Could you check a few things on this model? Use its own coordinates, in mm. A direction names the side the tool comes from. Coordinates: 2 decimals unless noted, no trailing zeros. Write each loop counter-clockwise with the first axis right and the second up, starting at its lowest first coordinate (ties: lowest second). Pieces come first, ordered by that corner, then holes.
Item 1: If I drill on probe 1 along Z at (x, y) = (0, 4.7); probe 2 along Z at (x, y) = (0, 6.45); probe 3 along X at (y, z) = (2.5, 12.5), over which ranges is the centre line in solid material (lowest first)?
Item 2: I want a section at B-B on y = 1.5. Please give me the cut outline in (x, z).
Item 3: I want a section at A-A on x = 13.5. Please give me the cut outline in (y, z), then the cut area to 3 significant figures.
Item 4: Thinking about a two-plate mould opening in Z: for faces 1 (the flat face through (0, 0, 6)), 2 (the cylindrical face through (23, 6, 0)), 3 (the cylindrical face through (18.5, 3.7, 2.4)), which applies, +Z half, -Z half, draft (parallel to the pull), parting line (faces both ways), or undercut?
Item 5: I want a section at D-D on x = 2.5. Please give me the cut outline in (y, z).
Item 6: For P1, Ø3, axis at x = 10.5, y = 1.5, coming from the +Z side; P2, Ø4, axis at x = 6, y = 5, coming from the +Z side; P3, Ø2, axis at x = -15, z = 17.5, coming from the +Y side; P4, Ø4, axis at x = 13, z = 8, coming from the -Y side, each with a flat end and sliding along its axis, tell me the tip position at first contact or that it passes through.
Item 7: I want a section at C-C on z = 4.5. Please give me the cut outline in (x, y).
Item 8: Which directions (+Z, -Z, +X, -X, +Y, -Y) give clear straight access to the entire face, cutting with the end or side of a thin tool? Please do faces 4 (the flat face through (24, 3.75, 2)), 5 (the flat face through (0, 4, -5)), 6 (the flat face through (13, 6.5, 8)), 7 (the flat face through (-24, 3.75, 2)).
from build123d import *

# Parameters (mm, degrees)
SZKIC2_R                    = 7.5
SZKIC2_R_2                  = 2.4
DODANIE_WYCI_GNI_CIE1_DEPTH = 3.75
SZKIC3_R                    = 5
DODANIE_WYCI_GNI_CIE2_DEPTH = 3.75
SZKIC9_R                    = 7.5
WYTNIJ_WYCI_GNI_CIE3_DEPTH  = 5
SZKIC10_R                   = 2.5
WYTNIJ_WYCI_GNI_CIE4_DEPTH  = 6.5


with BuildPart() as part:
    # Szkic2 → Dodanie-wyciągnięcie1 (new body)
    with BuildSketch(Plane(origin=(0, 0, 0), x_dir=(1, 0, 0), z_dir=(0, 1, 0))):
        with BuildLine():
            Line((-16, 5), (16, 5))
            ThreePointArc((16, 5), (24.235849057, -1.575471698), (17.660377358, -9.811320755))
            ThreePointArc((17.660377358, -9.811320755), (14.373605639, -12.807619738), (10, -12))
            Line((10, -12), (10, -14))
            ThreePointArc((10, -14), (0, -24), (-10, -14))
            Line((-10, -14), (-10, -12.057627201))
            ThreePointArc((-10, -12.057627201), (-14.369651741, -12.856788302), (-17.67794965, -9.892386213))
            ThreePointArc((-17.67794965, -9.892386213), (-24.285167931, -1.607218282), (-16, 5))
        make_face()
        with Locations(Location((0, -14, 0), (0, 0, 270))):
            Circle(SZKIC2_R, mode=Mode.SUBTRACT)
        with Locations(Location((-13, -8, 0), (0, 0, 270))):
            Circle(SZKIC2_R_2, mode=Mode.SUBTRACT)
        with Locations(Location((13, -8, 0), (0, 0, 270))):
            Circle(SZKIC2_R_2, mode=Mode.SUBTRACT)
        with BuildLine():
            Line((-16, 0), (16, 0))
            ThreePointArc((16, 0), (18.5, -2.5), (16, -5))
            Line((16, -5), (-16, -5))
            ThreePointArc((-16, -5), (-18.5, -2.5), (-16, 0))
        make_face(mode=Mode.SUBTRACT)
    extrude(amount=DODANIE_WYCI_GNI_CIE1_DEPTH)

    # Szkic3 → Dodanie-wyciągnięcie2 (add)
    with BuildSketch(Plane(origin=(0, 3.75, 0), x_dir=(1, 0, 0), z_dir=(0, 1, 0))):
        with BuildLine():
            Line((-16, 5), (16, 5))
            ThreePointArc((16, 5), (22.873192437, 0.342120663), (21.093817027, -7.76777683))
            Line((21.093817027, -7.76777683), (6.968542539, -21.17212764))
            ThreePointArc((6.968542539, -21.17212764), (0, -23.952289066), (-6.968542539, -21.17212764))
            Line((-6.968542539, -21.17212764), (-21.093817027, -7.76777683))
            ThreePointArc((-21.093817027, -7.76777683), (-22.873192437, 0.342120663), (-16, 5))
        make_face()
        with Locations(Location((0, -13.8, 0), (0, 0, 270))):
            Circle(SZKIC3_R, mode=Mode.SUBTRACT)
        with BuildLine():
            Line((-16, 0), (16, 0))
            ThreePointArc((16, 0), (18.5, -2.5), (16, -5))
            Line((16, -5), (-16, -5))
            ThreePointArc((-16, -5), (-18.5, -2.5), (-16, 0))
        make_face(mode=Mode.SUBTRACT)
    extrude(amount=DODANIE_WYCI_GNI_CIE2_DEPTH)

    # Szkic9 → Wytnij-wyciągnięcie3 (cut)
    with BuildSketch(Plane.XZ):
        with Locations(Location((0, 14, 0), (0, 0, 270))):
            Circle(SZKIC9_R)
    extrude(amount=-WYTNIJ_WYCI_GNI_CIE3_DEPTH, mode=Mode.SUBTRACT)

    # Szkic10 → Wytnij-wyciągnięcie4 (cut)
    with BuildSketch(Plane.XZ):
        with Locations(Location((-13, 8, 0), (0, 0, 270))):
            Circle(SZKIC10_R)
        with Locations(Location((13, 8, 0), (0, 0, 270))):
            Circle(SZKIC10_R)
    extrude(amount=-WYTNIJ_WYCI_GNI_CIE4_DEPTH, mode=Mode.SUBTRACT)


solid = part.part
Response values:
1. probe 1: z = -5 to 0, 5 to 6.5, 21.5 to 23.95
1. probe 2: z = -5 to 0, 5 to 8.8, 18.8 to 23.95
1. probe 3: x = -15.28 to -10.72, -10 to -7.35, 7.35 to 10, 10.82 to 15.18
2. outline: (-17.68, 9.89) arc R7.49 ccw to (-16, -5) - (16, -5) arc R7.45 ccw to (17.66, 9.81) arc R5 ccw to (10, 12) - (10, 14) arc R10 ccw to (-10, 14) - (-10, 12.06) arc R5.05 ccw to start; hole (-16, 0) - (16, 0) arc R2.5 ccw to (16, 5) - (-16, 5) arc R2.5 ccw to start; hole circle Ø5 at (-13, 8); hole circle Ø15 at (0, 14); hole circle Ø5 at (13, 8)
3. outline: (0, -5) - (7.5, -5) - (7.5, 0) - (0, 0) - close; (0, 5) - (7.5, 5) - (7.5, 14.97) - (3.75, 14.97) - (3.75, 12.97) - (0, 12.97) - (0, 10.45) - (6.5, 10.45) - (6.5, 5.55) - (0, 5.55) - close
3. area: 73.0 mm2
4. face 1: draft
4. face 2: parting line
4. face 3: undercut
5. outline: (0, -5) - (7.5, -5) - (7.5, 0) - (0, 0) - close; (0, 5) - (7.5, 5) - (7.5, 9.47) - (5, 9.47) - (5, 6.93) - (0, 6.93) - close; (0, 21.07) - (5, 21.07) - (5, 18.13) - (7.5, 18.13) - (7.5, 23.64) - (3.75, 23.64) - (3.75, 23.68) - (0, 23.68) - close
6. P1: stops at z = 18.36
6. P2: stops at z = 23.13
6. P3: passes through
6. P4: stops at y = 6.5
7. outline: (-24.05, 0) - (-17.5, 0) - (-17.5, 7.5) - (-23.1, 7.5) - (-23.1, 3.75) - (-24.05, 3.75) - close; (17.5, 0) - (23.98, 0) - (23.98, 3.75) - (23.1, 3.75) - (23.1, 7.5) - (17.5, 7.5) - close
8. face 4: +X, +Y
8. face 5: -Z, +Y, -Y
8. face 6: -Y
8. face 7: -X, +Y
